Can you work these out from the model? Positions are in its coordinate system, mm. Face numbers are marked on the shaded views. A direction names the side the tool comes from. Coordinates: 2 decimals unless noted, no trailing zeros. Order: outer loops, then holes, each group sorted by start corner. A loop starts at its lowest first (then second) coordinate and runs counter-clockwise, first axis right, second up. Notation, with made-up numbers: (-10.5, 10.5) - (-4.5, 10.5) arc R19 ccw to (-4.5, 38.5) - close; hole circle Ø9 at (-27, -29.75). An arc over 180 degrees is marked (long way). Return JSON: item names as keys, results as strings. Group by question number.
1) For pin 1 Ø2 at (x, z) = (4.5, 24.5) entering from -Y; pin 2 Ø5 at (x, z) = (-2.5, 45.5) entering from -Y; pin 3 Ø5 at (x, y) = (-7, -5) entering from +Z, each with a flat end and sliding along its axis, tell me the tip position at first contact or that it passes through.
2) If I drill on line 1 along Y through (x, z) = (0, 58.5); line 2 along Y through (x, z) = (0, 21); line 3 along Z through (x, y) = (-0.5, 2.25), over which ranges is the centre line in solid material (lowest first)?
3) Imagine slicing it at A-A (z = 11). Write out the boundary of the cut face in (x, y).
4) Which directions (+Z, -Z, +X, -X, +Y, -Y) give clear straight access to the entire face, cutting with the end or side of a thin tool? Please do the marked faces 1 and 2.
Solid Edge part; units mm, degrees
sketch "Sketch1" plane through (0, 0, 0) normal (0, 0, 1) x (1, 0, 0)
  circle A0 centre (0, 0) radius 9
extrude "Protrusion1" add sketch "Sketch1" along normal blind 63
sketch "Sketch2" plane through (0, 0, 0) normal (0, -1, 0) x (1, 0, 0)
  line L0 (12.5226, 43) -> (12.5226, 68.3546)
  line L1 (12.5226, 68.3546) -> (3, 68.3546)
  line L2 (3, 68.3546) -> (3, 63)
  line L3 (3, 63) -> (3, 58)
  spline S0 degree 3 poles (3, 58) (2.984, 54.7412) (4.2657, 49.2147) (8.5336, 46.9653) (8.8514, 44.0312) (9, 43) knots 0 0 0 0 0.509409 0.837698 1 1 1 1
  line L4 (9, 43) -> (12.5226, 43)
revolve "RevolvedCutout1" cut sketch "Sketch2" angle 360 about axis through (0, 0, 43.0463) along (0, 0, 1)
shell "Thinwall_1" thickness 4 removed faces 0 other thickness 2 on face (4.9805, 7.4963, 35.4033) other thickness 2 on face (1.6602, 2.4988, 62.1167)
sketch "Sketch3" plane through (0, 0, 63) normal (0, 0, 1) x (1, 0, 0)
  circle A0 centre (0, 0) radius 2
extrude "ExtrudedCutout_1" cut sketch "Sketch3" against normal blind 47.9511
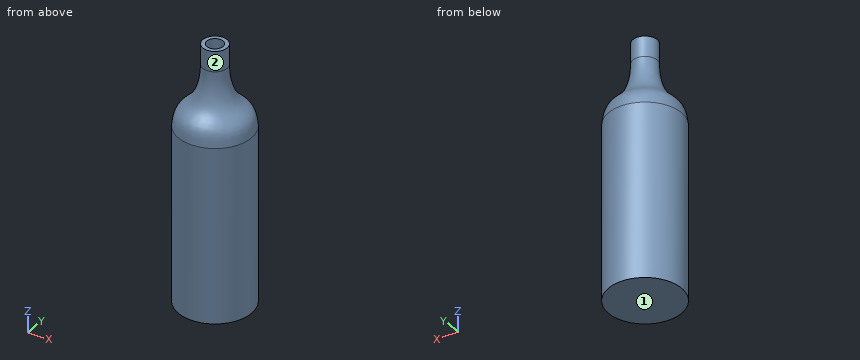
Calculated:
{
 "1": {"pin 1": "y = -8.29", "pin 2": "y = -8.87", "pin 3": "z = 48.6"},
 "2": {"line 1": "-3 to -2, 2 to 3", "line 2": "-9 to -7, 7 to 9", "line 3": "0 to 4, 50.74 to 63"},
 "3": {"outline": "circle Ø18 at (0, 0); hole circle Ø14 at (0, 0)"},
 "4": {"face 1": "-Z, +X, -X, +Y, -Y", "face 2": "+Z"}
}
